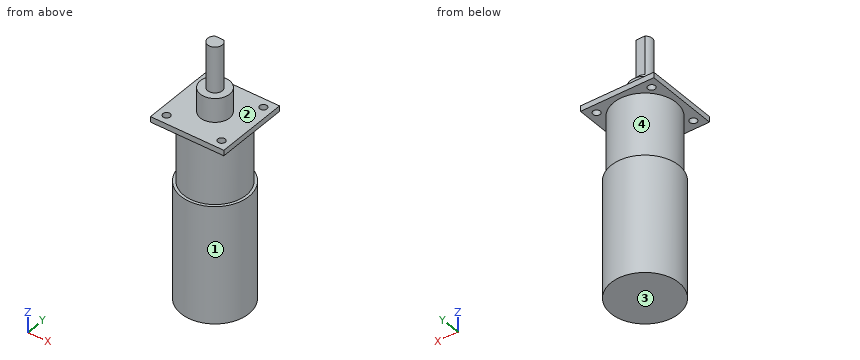
Autodesk Inventor part; units mm, degrees
ref_plane "YZ Plane" through (0, 0, 0) normal (1, 0, 0) x (0, 1, 0)
ref_plane "XZ Plane" through (0, 0, 0) normal (0, 1, 0) x (-1, 0, 0)
ref_plane "XY Plane" through (0, 0, 0) normal (0, 0, 1) x (1, 0, 0)
sketch "Sketch1" plane through (0, 0, 0) normal (0, 0, 1) x (1, 0, 0)
  line L0 (0, 0) -> (40, 0)
  line L1 (40, 0) -> (40, 40)
  line L2 (40, 40) -> (0, 40)
  line L3 (0, 40) -> (0, 0)
  dimension "d0" = 40
  dimension "d1" = 40
extrude "Extrusion1" add sketch "Sketch1" along normal blind 3
sketch "Sketch2" plane through (0, 0, 3) normal (0, 0, 1) x (1, 0, 0)
  line L0 (40, 0) -> (0, 0)
  line L1 (40, 40) -> (40, 0)
  line L2 (35, 5) -> (5, 5)
  line L3 (5, 5) -> (5, 35)
  line L4 (5, 35) -> (35, 35)
  line L5 (35, 35) -> (35, 5)
  circle A0 centre (20, 20) radius 8
  dimension "d4" = 30
  dimension "d5" = 30
  dimension "d6" = 5
  dimension "d7" = 5
  dimension "d8" = 16
extrude "Extrusion2" add sketch "Sketch2" along normal blind 13 contours A0
sketch "Sketch3" plane through (0, 0, 3) normal (0, 0, 1) x (1, 0, 0)
  line L0 (40, 0) -> (0, 0)
  line L1 (40, 40) -> (40, 0)
  line L2 (5, 5) -> (35, 5)
  line L3 (35, 5) -> (35, 35)
  line L4 (35, 35) -> (5, 35)
  line L5 (5, 35) -> (5, 5)
  dimension "d11" = 30
  dimension "d12" = 30
  dimension "d13" = 5
  dimension "d14" = 5
hole "Hole1" at (5, 5, 3) at (35, 5, 3) at (35, 35, 3) at (5, 35, 3) direction (0, 0, -1) diameter 4 end through all
sketch "Sketch4" plane through (20, 20, 16) normal (0, 0, 1) x (1, 0, 0)
  circle A0 centre (0, 0) radius 8
  circle A1 centre (0, 0) radius 4
  point P0 (-20, -20)
  dimension "d22" = 8
extrude "Extrusion3" add sketch "Sketch4" along normal blind 25 contours A1
sketch "Sketch5" plane through (20, 20, 41) normal (0, 0, 1) x (1, 0, 0)
  circle A0 centre (0, 0) radius 4
  line L0 (-4, 0) -> (4, 0)
  line L1 (4, 0) -> (4, 4)
  line L2 (4, 4) -> (-4, 4)
  line L3 (-4, 4) -> (-4, 0)
  line L4 (-4, 4) -> (4, 4)
  line L5 (4, 4) -> (4, 3.2)
  line L6 (4, 3.2) -> (-4, 3.2)
  line L7 (-4, 3.2) -> (-4, 4)
  point P0 (-20, -20)
  dimension "d25" = 0.8
extrude "Extrusion4" cut sketch "Sketch5" against normal blind 21 contours L6 L3 L2 A0 | A0 L6 | A0 L2 L1 L6
sketch "Sketch6" plane through (0, 0, 0) normal (0, 0, -1) x (-1, 0, 0)
  circle A0 centre (-20, 20) radius 17
  dimension "d28" = 34
extrude "Extrusion5" add sketch "Sketch6" along normal blind 35
sketch "Sketch7" plane through (20, 20, -35) normal (0, 0, -1) x (-1, 0, 0)
  circle A0 centre (0, 0) radius 17
  circle A1 centre (0, 0) radius 18.5
  point P0 (20, -20)
  dimension "d31" = 37
extrude "Extrusion6" add sketch "Sketch7" along normal blind 64 contours A0 | A1
properties part number "mr85vel 3 etapas" material "UHMW, White"
Design review of the part built by this model. Coordinates are the model's own, in mm. Face numbers are marked on the shaded views. Give positions to 0.01 mm unless a question says otherwise; leave off trailing zeros. Write each loop counter-clockwise with the first axis right and the second up, starting at its lowest first coordinate (ties: lowest second). Pieces come first, ordered by that corner, then holes.
(1) Add section B-B (x = 5). Give the boundary of the cut face in (y, z), and give its area (3 significant figures).
Checked values:
outline: (0, 0) - (3, 0) - (3, 3) - (0, 3) - close; (7, 0) - (12, 0) - (12, -35) - (9.17, -35) - (9.17, -99) - (30.83, -99) - (30.83, -35) - (28, -35) - (28, 0) - (33, 0) - (33, 3) - (7, 3) - close; (37, 0) - (40, 0) - (40, 3) - (37, 3) - close
area: 2,040 mm2
(2) Add section A-A (y = 20). Give the boundary of the cut face in (x, z).
Checked values:
outline: (0, 0) - (3, 0) - (3, -35) - (1.5, -35) - (1.5, -99) - (38.5, -99) - (38.5, -35) - (37, -35) - (37, 0) - (40, 0) - (40, 3) - (28, 3) - (28, 16) - (24, 16) - (24, 41) - (16, 41) - (16, 16) - (12, 16) - (12, 3) - (0, 3) - close
(3) Clearance check with flat-ended pins moving along their axes: pin 1 Ø1.5 at (y, z) = (16.5, 7) entering from +X; pin 2 Ø4 at (x, z) = (27, -39.5) entering from -Y; pin 3 Ø6 at (x, z) = (7.5, -81.5) entering from +Y. State where each tip first meets the part, or that it passes through.
Checked values:
pin 1: stops at x = 27.51
pin 2: stops at y = 2.19
pin 3: stops at y = 35.87
(4) Wall thickness on line 1 along X through (y, z) = (35, 1); line 2 along Z through (x, y) = (9, 7); line 3 along Z through (x, y) = (28, 30.5): over which ranges is each line inside the solid? List them lowest first.
Checked values:
line 1: x = 0 to 3, 7 to 33, 37 to 40
line 2: z = -99 to -35, 0 to 3
line 3: z = -99 to 3
(5) Add section D-D (x = 20). Give the boundary of the cut face in (y, z).
Checked values:
outline: (0, 0) - (3, 0) - (3, -35) - (1.5, -35) - (1.5, -99) - (38.5, -99) - (38.5, -35) - (37, -35) - (37, 0) - (40, 0) - (40, 3) - (28, 3) - (28, 16) - (24, 16) - (24, 20) - (23.2, 20) - (23.2, 41) - (16, 41) - (16, 16) - (12, 16) - (12, 3) - (0, 3) - close
(6) Mouldability with a two-part tool opening along Z and no side actions: class the marked faces 1, 2, 3 and 4 as +Z half, -Z half, draft (parallel to the pull), parting line (faces both ways), or undercut.
Checked values:
face 1: draft
face 2: +Z half
face 3: -Z half
face 4: undercut
